from build123d import *

# Parameters (mm, degrees)
F0_W          = 14
F0_H          = 6
F0_W_2        = 10
F0_H_2        = 2
F1_DEPTH      = 15
F2_W          = 24
F2_H          = 24
F3_DEPTH      = 4
F3_DEPTH_BACK = 2
F5_D          = 18
F6_R          = 2
F7_D          = 2.2606
F7_DEPTH      = 2.3
F7_TIP        = 0.6791527577


with BuildPart() as f1:
    # F0 (on Front) → F1 (new body)
    with BuildSketch(Plane.XZ):
        with Locations((0, 1)):
            Rectangle(F0_W, F0_H)
        with Locations((0, 1)):
            Rectangle(F0_W_2, F0_H_2, mode=Mode.SUBTRACT)
    extrude(amount=F1_DEPTH)

    # F2 (on Top) → F3 (join, two sides)
    with BuildSketch(Plane.XY) as f3_sk:
        with Locations((0, -27)):
            Rectangle(F2_W, F2_H)
    extrude(amount=F3_DEPTH)
    extrude(f3_sk.sketch, amount=-F3_DEPTH_BACK)

    # F5 (through all)
    with Locations(Plane(origin=(0, 0, -2), x_dir=(1, 0, 0), z_dir=(0, 0, -1))):
        with Locations((0, 27)):
            Hole(F5_D / 2)

    # F6
    f6_edges = [f1.edges().sort_by_distance(p)[0] for p in [
        (12, -39, 1),
        (12, -15, 1),
        (7, -15, 1),
        (-12, -39, 1),
        (-12, -15, 1),
        (-7, -15, 1),
    ]]
    fillet(f6_edges, radius=F6_R)

    # F7
    with Locations(Plane(origin=(0, 0, -2), x_dir=(1, 0, 0), z_dir=(0, 0, -1))):
        with Locations((0, 7.5)):
            Hole(F7_D / 2, depth=F7_DEPTH)
            with Locations((0, 0, -(F7_DEPTH + F7_TIP / 2))):  # 118° drill point
                Cone(0, F7_D / 2, F7_TIP, mode=Mode.SUBTRACT)


solid = f1.part
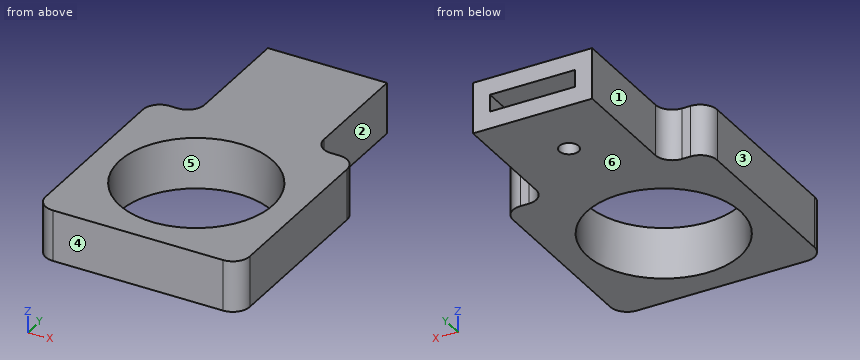
Model file for the job. Use its own axes, mm. Face numbers are marked on the shaded views. A direction names the side the tool comes from. Round coordinates to 2 decimals unless told otherwise and drop trailing zeros. Order: outer loops, then holes, each group sorted by start corner. A loop starts at its lowest first (then second) coordinate and runs counter-clockwise, first axis right, second up.
(1) Band-saw the part on C-C (z = 0.95). List the corners of the cut face in (x, y).
(2) Drill centre lines: line 1 (Y direction, x = 0, z = -1); line 2 (X direction, y = -7.5, z = -0.4); line 3 (Y direction, x = 0, z = 0.1). Where is each one in solid material? Low to high.
(3) Band-saw the part on B-B (y = -27). List the corners of the cut face in (x, z), then the cut area to 3 significant figures.
(4) Pull direction Y, two halves, no side cores. Call the marked faces 4, 5 and 6: released by +Y, released by -Y, zero draft, split by the parting line, or undercut.
(5) Band-saw the part on A-A (x = 0). List the corners of the cut face in (y, z).
(6) 3-axis set-ups, long thin cutter, end or side, ignore diameter. For the marked faces 1, 2 and 3: which of +Z, -Z, +X, -X, +Y, -Y reach the whole face in a straight line?
(7) Pin check, flat tips, straight feed: pin 1 (3 mm diameter, centred on y = -9, z = 0, fed in from +X); pin 2 (1 mm diameter, centred on y = -7.5, z = 1, fed in from -X); pin 3 (1 mm diameter, centred on x = 2, z = 1, fed in from +Y). Stop position of each tip, or through.
(8) Band-saw the part on D-D (x = -8). List the corners of the cut face in (y, z), then the cut area to 3 significant figures.
Verdict:
1. outline: (-12, -37) arc R2 ccw to (-10, -39) - (10, -39) arc R2 ccw to (12, -37) - (12, -17) arc R2 ccw to (10, -15) - (9, -15) arc R2 cw to (7, -13) - (7, 0) - (5, 0) - (5, -15) - (-5, -15) - (-5, 0) - (-7, 0) - (-7, -13) arc R2 cw to (-9, -15) - (-10, -15) arc R2 ccw to (-12, -17) - close; hole circle Ø18 at (0, -27)
2. line 1: y = -39 to -36, -18 to -8.63, -6.37 to 0
2. line 2: x = -7 to -1.13, 1.13 to 7
2. line 3: y = -39 to -36, -18 to -15
3. outline: (-12, -2) - (-9, -2) - (-9, 4) - (-12, 4) - close; (9, -2) - (12, -2) - (12, 4) - (9, 4) - close
3. area: 36.0 mm2
4. face 4: released by -Y
4. face 5: undercut
4. face 6: zero draft
5. outline: (-39, -2) - (-36, -2) - (-36, 4) - (-39, 4) - close; (-18, -2) - (-8.63, -2) - (-8.63, 0) - (-15, 0) - (-15, 2) - (0, 2) - (0, 4) - (-18, 4) - close; (-6.37, -2) - (0, -2) - (0, 0) - (-6.37, 0) - close
6. face 1: +Z, -Z, -X, +Y
6. face 2: +Z, -Z, +X, +Y
6. face 3: +Z, -Z, -X, +Y, -Y
7. pin 1: stops at x = 7
7. pin 2: stops at x = -7
7. pin 3: stops at y = -15
8. outline: (-39, -2) - (-31.12, -2) - (-31.12, 4) - (-39, 4) - close; (-22.88, -2) - (-14.73, -2) - (-14.73, 4) - (-22.88, 4) - close
8. area: 96.1 mm2
